Can you work these out from the model? Positions are in its coordinate system, mm. Face numbers are marked on the shaded views. A direction names the side the tool comes from. Coordinates: 2 decimals unless noted, no trailing zeros. Loops run counter-clockwise (first coordinate to the right, second up) from the corner with the lowest first, then second, coordinate; pieces in that order, holes last. Notation, with made-up numbers: M 46.25,87 L 89.25,87 A21 ccw 89.25,121 Z; hole C 30,0.5 d7. An arc over 180 degrees is marked long. Return JSON: item names as keys, results as strings. Group by question number.
```python
from build123d import *

# Parameters (mm, degrees)
SKETCH1_W            = 93
SKETCH1_H            = 100
BOSS_EXTRUDE2_DEPTH  = 10
SKETCH4_W            = 10.01
SKETCH4_H            = 15
BOSS_EXTRUDE4_DEPTH  = 24
SKETCH5_R            = 2
CUT_EXTRUDE1_DEPTH   = 50
SKETCH7_R            = 11
CUT_EXTRUDE3_DEPTH   = 50
SKETCH14_W           = 61.5
SKETCH14_H           = 42
CUT_EXTRUDE8_DEPTH   = 4
SKETCH19_R           = 11
CUT_EXTRUDE11_DEPTH  = 15
SKETCH20_R           = 2
CUT_EXTRUDE12_DEPTH  = 10
SKETCH21_W           = 40
SKETCH21_H           = 6
BOSS_EXTRUDE5_DEPTH  = 27
SKETCH22_W           = 40
SKETCH22_H           = 6.3
BOSS_EXTRUDE7_DEPTH  = 40
SKETCH23_R           = 8
CUT_EXTRUDE13_DEPTH  = 40
SKETCH24_W           = 118.277817783
SKETCH24_H           = 41.8
CUT_EXTRUDE14_DEPTH  = 40
SKETCH25_W           = 31.5
SKETCH25_H           = 23.2
CUT_EXTRUDE15_DEPTH  = 20
CUT_EXTRUDE18_DEPTH  = 3
SKETCH27_R           = 4.1
SKETCH27_R_2         = 4
CUT_EXTRUDE29_DEPTH  = 3
SKETCH28_W           = 29.5
SKETCH28_H           = 58.2
CUT_EXTRUDE30_DEPTH  = 23
SKETCH29_W           = 32
SKETCH29_H           = 4
CUT_EXTRUDE31_DEPTH  = 23
SKETCH31_W           = 32
SKETCH31_H           = 6
BOSS_EXTRUDE9_DEPTH  = 6.6
SKETCH32_W           = 32
SKETCH32_H           = 6
BOSS_EXTRUDE10_DEPTH = 10
SKETCH33_R           = 2
CUT_EXTRUDE32_DEPTH  = 10
BOSS_EXTRUDE11_START = -32
BOSS_EXTRUDE11_DEPTH = 32
SKETCH35_R           = 3.5
CUT_EXTRUDE33_DEPTH  = 10
SKETCH36_W           = 27
SKETCH36_H           = 46
CUT_EXTRUDE34_DEPTH  = 50
SKETCH38_W           = 31.75
SKETCH38_H           = 35
CUT_EXTRUDE35_DEPTH  = 50
SKETCH40_W           = 4
SKETCH40_H           = 77.818306413
CUT_EXTRUDE37_DEPTH  = 110
SKETCH41_W           = 28
SKETCH41_H           = 1.72
CUT_EXTRUDE38_DEPTH  = 50


with BuildPart() as part:
    # Sketch1 → Boss-Extrude2 (new body)
    with BuildSketch(Plane.XY):
        with Locations((-29.68705036, 14.928057554)):
            Rectangle(SKETCH1_W, SKETCH1_H)
    extrude(amount=BOSS_EXTRUDE2_DEPTH)

    # Sketch4 → Boss-Extrude4 (add)
    with BuildSketch(Plane(origin=(16.81294964, 0, 0), x_dir=(0, 0, -1), z_dir=(1, 0, 0))):
        with Locations((-4.995, -12.571942446)):
            Rectangle(SKETCH4_W, SKETCH4_H)
    extrude(amount=BOSS_EXTRUDE4_DEPTH)

    # Sketch5 → Cut-Extrude1 (cut)
    with BuildSketch(Plane(origin=(0, -5.071942446, 0), x_dir=(1, 0, 0), z_dir=(0, 1, 0))):
        with Locations(Location((26.81294964, -5, 0), (0, 0, 180))):
            Circle(SKETCH5_R)
    extrude(amount=-CUT_EXTRUDE1_DEPTH, mode=Mode.SUBTRACT)

    # Sketch7 → Cut-Extrude3 (cut)
    with BuildSketch(Plane(origin=(0, 0, 0), x_dir=(-1, 0, 0), z_dir=(0, 0, -1))):
        with Locations((24.18705036, 36.928057554)):
            Circle(SKETCH7_R)
    extrude(amount=-CUT_EXTRUDE3_DEPTH, mode=Mode.SUBTRACT)

    # Sketch14 → Cut-Extrude8 (cut)
    with BuildSketch(Plane.XY.offset(10)):
        with Locations((-13.93705036, 36.789132279)):
            Rectangle(SKETCH14_W, SKETCH14_H)
    extrude(amount=-CUT_EXTRUDE8_DEPTH, mode=Mode.SUBTRACT)

    # Sketch19 → Cut-Extrude11 (cut)
    with BuildSketch(Plane(origin=(0, 0, 0), x_dir=(-1, 0, 0), z_dir=(0, 0, -1))):
        with Locations((53.18705036, 36.928057554)):
            Circle(SKETCH19_R)
    extrude(amount=-CUT_EXTRUDE11_DEPTH, mode=Mode.SUBTRACT)

    # Sketch20 → Cut-Extrude12 (cut)
    with BuildSketch(Plane.XY.offset(6)):
        with Locations((-34.68705036, 50.928057554)):
            Circle(SKETCH20_R)
        with Locations((5.31294964, 50.928057554)):
            Circle(SKETCH20_R)
        with Locations((-34.68705036, 22.928057554)):
            Circle(SKETCH20_R)
        with Locations((5.31294964, 22.928057554)):
            Circle(SKETCH20_R)
    extrude(amount=-CUT_EXTRUDE12_DEPTH, mode=Mode.SUBTRACT)

    # Sketch21 → Boss-Extrude5 (add)
    with BuildSketch(Plane(origin=(0, 0, 0), x_dir=(-1, 0, 0), z_dir=(0, 0, -1))):
        with Locations((56.18705036, 61.928057554)):
            Rectangle(SKETCH21_W, SKETCH21_H)
    extrude(amount=BOSS_EXTRUDE5_DEPTH)

    # Sketch22 → Boss-Extrude7 (add)
    with BuildSketch(Plane.XZ.offset(-58.928057554)):
        with Locations((-56.18705036, -23.85)):
            Rectangle(SKETCH22_W, SKETCH22_H)
    extrude(amount=BOSS_EXTRUDE7_DEPTH)

    # Sketch23 → Cut-Extrude13 (cut)
    with BuildSketch(Plane.XY.offset(10)):
        with Locations((-53.18705036, 36.928057554)):
            Circle(SKETCH23_R)
    extrude(amount=-CUT_EXTRUDE13_DEPTH, mode=Mode.SUBTRACT)

    # Sketch24 → Cut-Extrude14 (cut)
    with BuildSketch(Plane.XY.offset(10)):
        with Locations((-17.048141468, -14.171942446)):
            Rectangle(SKETCH24_W, SKETCH24_H)
    extrude(amount=-CUT_EXTRUDE14_DEPTH, mode=Mode.SUBTRACT)

    # Sketch25 → Cut-Extrude15 (cut)
    with BuildSketch(Plane.XY.offset(10)):
        with Locations((-60.43705036, 18.328057554)):
            Rectangle(SKETCH25_W, SKETCH25_H)
    extrude(amount=-CUT_EXTRUDE15_DEPTH, mode=Mode.SUBTRACT)

    # Sketch26 → Cut-Extrude18 (cut)
    with BuildSketch(Plane.XY.offset(6)):
        with BuildLine():
            Line((14.30212304, 57.789132279), (6.863398886, 57.789132279))
            Line((6.863398886, 57.789132279), (6.863398886, 54.615347499))
            ThreePointArc((6.863398886, 54.615347499), (8.24773413, 53.645968516), (9.108195728, 52.191428892))
            Line((9.108195728, 52.191428892), (14.30212304, 52.191428892))
            Line((14.30212304, 52.191428892), (14.30212304, 57.789132279))
        make_face()
        with BuildLine():
            Line((6.863398886, 19.240767609), (6.863398886, 15.789132279))
            Line((6.863398886, 15.789132279), (14.30212304, 15.789132279))
            Line((14.30212304, 15.789132279), (14.30212304, 20.928057554))
            Line((14.30212304, 20.928057554), (8.777051255, 20.928057554))
            ThreePointArc((8.777051255, 20.928057554), (7.95835451, 19.927752057), (6.863398886, 19.240767609))
        make_face()
        with BuildLine():
            Line((-36.237499605, 57.789132279), (-44.68705036, 57.789132279))
            Line((-44.68705036, 57.789132279), (-44.68705036, 52.191428892))
            Line((-44.68705036, 52.191428892), (-38.482296447, 52.191428892))
            ThreePointArc((-38.482296447, 52.191428892), (-37.621834849, 53.645968516), (-36.237499605, 54.615347499))
            Line((-36.237499605, 54.615347499), (-36.237499605, 57.789132279))
        make_face()
        with BuildLine():
            Line((-44.68705036, 21.664686216), (-44.68705036, 15.789132279))
            Line((-44.68705036, 15.789132279), (-36.237499605, 15.789132279))
            Line((-36.237499605, 15.789132279), (-36.237499605, 19.240767609))
            ThreePointArc((-36.237499605, 19.240767609), (-37.621834849, 20.210146592), (-38.482296447, 21.664686216))
            Line((-38.482296447, 21.664686216), (-44.68705036, 21.664686216))
        make_face()
    extrude(amount=-CUT_EXTRUDE18_DEPTH, mode=Mode.SUBTRACT)

    # Sketch27 → Cut-Extrude29 (cut)
    with BuildSketch(Plane.XY.offset(6)):
        with Locations((5.31294964, 50.928057554)):
            Circle(SKETCH27_R)
        with Locations((5.31294964, 22.928057554)):
            Circle(SKETCH27_R_2)
        with Locations((-34.68705036, 50.928057554)):
            Circle(SKETCH27_R)
        with Locations((-34.68705036, 22.928057554)):
            Circle(SKETCH27_R)
    extrude(amount=-CUT_EXTRUDE29_DEPTH, mode=Mode.SUBTRACT)

    # Sketch28 → Cut-Extrude30 (cut)
    with BuildSketch(Plane(origin=(0, 0, 0), x_dir=(-1, 0, 0), z_dir=(0, 0, -1))):
        with Locations((-2.06294964, 35.828057554)):
            Rectangle(SKETCH28_W, SKETCH28_H)
    extrude(amount=-CUT_EXTRUDE30_DEPTH, mode=Mode.SUBTRACT)

    # Sketch29 → Cut-Extrude31 (cut)
    with BuildSketch(Plane(origin=(0, 15.789132279, 0), x_dir=(1, 0, 0), z_dir=(0, 1, 0))):
        with Locations((-28.68705036, -8)):
            Rectangle(SKETCH29_W, SKETCH29_H)
    extrude(amount=-CUT_EXTRUDE31_DEPTH, mode=Mode.SUBTRACT)

    # Sketch31 → Boss-Extrude9 (add)
    with BuildSketch(Plane.XZ.offset(-6.728057554)):
        with Locations((-28.68705036, 3)):
            Rectangle(SKETCH31_W, SKETCH31_H)
    extrude(amount=BOSS_EXTRUDE9_DEPTH)

    # Sketch32 → Boss-Extrude10 (add)
    with BuildSketch(Plane.XY.offset(6)):
        with Locations((-28.68705036, 3.128057554)):
            Rectangle(SKETCH32_W, SKETCH32_H)
    extrude(amount=BOSS_EXTRUDE10_DEPTH)

    # Sketch33 → Cut-Extrude32 (cut)
    with BuildSketch(Plane(origin=(0, 6.128057554, 0), x_dir=(1, 0, 0), z_dir=(0, 1, 0))):
        with Locations(Location((-33.68705036, -11, 0), (0, 0, 270))):
            Circle(SKETCH33_R)
        with Locations(Location((-19.68705036, -11, 0), (0, 0, 270))):
            Circle(SKETCH33_R)
    extrude(amount=-CUT_EXTRUDE32_DEPTH, mode=Mode.SUBTRACT)

    # Sketch34 → Boss-Extrude11 (add)
    with BuildSketch(Plane(origin=(-12.68705036, 0, 0), x_dir=(0, 0, -1), z_dir=(1, 0, 0)).offset(BOSS_EXTRUDE11_START)):
        Polygon((-16, 6.128057554), (-6, 6.128057554), (-6, 14.058360342), align=None)
    extrude(amount=BOSS_EXTRUDE11_DEPTH)

    # Sketch35 → Cut-Extrude33 (cut)
    with BuildSketch(Plane.XZ.offset(-6.128057554)):
        with Locations((-19.68705036, 11)):
            Circle(SKETCH35_R)
        with Locations((-33.68705036, 11)):
            Circle(SKETCH35_R)
    extrude(amount=-CUT_EXTRUDE33_DEPTH, mode=Mode.SUBTRACT)

    # Sketch36 → Cut-Extrude34 (cut)
    with BuildSketch(Plane(origin=(-36.18705036, 0, 0), x_dir=(0, 0, -1), z_dir=(1, 0, 0))):
        with Locations((13.5, 41.928057554)):
            Rectangle(SKETCH36_W, SKETCH36_H)
    extrude(amount=-CUT_EXTRUDE34_DEPTH, mode=Mode.SUBTRACT)

    # Sketch38 → Cut-Extrude35 (cut)
    with BuildSketch(Plane.XY.offset(10)):
        with Locations((-60.31205036, 47.428057554)):
            Rectangle(SKETCH38_W, SKETCH38_H)
    extrude(amount=-CUT_EXTRUDE35_DEPTH, mode=Mode.SUBTRACT)

    # Sketch40 → Cut-Extrude37 (cut)
    with BuildSketch(Plane.XY.offset(16)):
        with Locations((-42.68705036, 39.037210761)):
            Rectangle(SKETCH40_W, SKETCH40_H)
    extrude(amount=-CUT_EXTRUDE37_DEPTH, mode=Mode.SUBTRACT)

    # Sketch41 → Cut-Extrude38 (cut)
    with BuildSketch(Plane.XY.offset(16)):
        with Locations((-26.68705036, 0.988057554)):
            Rectangle(SKETCH41_W, SKETCH41_H)
    extrude(amount=-CUT_EXTRUDE38_DEPTH, mode=Mode.SUBTRACT)


solid = part.part
```
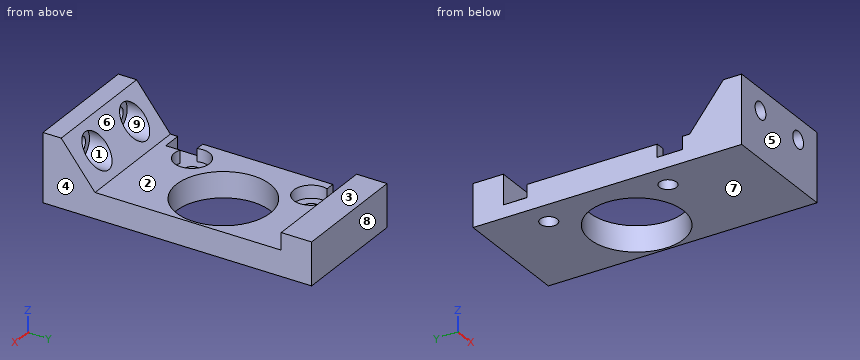
1) For the marked faces 1, 2, 3, 4 and 5, which set-ups out of +Z, -Z, +X, -X, +Y, -Y let a thin tool reach every point of the face, with its end or its side?
2) Suppose I cut it at C-C, the plane z = 8.25. List the corners of the cut face in (x, y) for me.
3) For pin 1 (8 mm diameter, centred on x = -37.5, y = 22.5, fed in from +Z); pin 2 (2.5 mm diameter, centred on x = -34.69, y = 50.93, fed in from +Z); pin 3 (0.9 mm diameter, centred on y = 17.5, z = 4.5, fed in from -X); pin 4 (5.5 mm diameter, centred on x = -30, y = 62, fed in from +Z), each with a flat end and sliding along its axis, tell me the tip position at first contact or that it passes through.
4) Suppose I cut it at A-A, the plane y = 41. List the corners of the cut face in (x, z) for me, then the cut area to 3 significant figures.
5) If I drill on line 1 (X direction, y = 3.3, z = 11); line 2 (Y direction, x = -36.5, z = 1.75); line 3 (Z direction, x = -36.75, y = 33), over which ranges is the centre line in solid material (lowest first)? Write a range as from..to.
6) If we mould it in two halves opening along Z, with no side actions, what happens to the marked faces 6, 7, 8 and 9? For each: +Z half, -Z half, draft (parallel to the pull), parting line (faces both ways), or undercut.
7) Suppose I cut it at D-D, the plane z = 11. List the corners of the cut face in (x, y) for me, then the cut area to 3 significant figures.
8) Suppose I cut it at B-B, the plane x = -27.75. List the corners of the cut face in (y, z) for me.
Returned:
{
 "1": {"face 1": "none", "face 2": "+Z, +X, -X", "face 3": "+Z, +X, -X, +Y", "face 4": "+Z, -Z, +X, +Y, -Y", "face 5": "+Z, -Z, +X, -X, -Y"},
 "2": {"outline": "M -40.69,1.85 L -12.69,1.85 L -12.69,12.27 L -17.52,12.27 L -17.52,6.13 L -21.85,6.13 L -21.85,12.27 L -31.52,12.27 L -31.52,6.13 L -35.85,6.13 L -35.85,12.27 L -40.69,12.27 Z; M -40.69,57.79 L -12.69,57.79 L -12.69,64.93 L -40.69,64.93 Z"},
 "3": {"pin 1": "stops at z = 6", "pin 2": "passes through", "pin 3": "stops at x = -36.24", "pin 4": "stops at z = 10"},
 "4": {"outline": "M -40.69,0 L -34.41,0 L -34.41,6 L -40.69,6 Z; M -13.97,0 L -12.69,0 L -12.69,6 L -13.97,6 Z", "area": "45.4 mm²"},
 "5": {"line 1": "x = -40.69..-35.69, -31.69..-21.69, -17.69..-12.69", "line 2": "y = 1.85..22.08, 23.77..50.08, 51.77..64.93", "line 3": "z = 0..6"},
 "6": {"face 6": "+Z half", "face 7": "-Z half", "face 8": "draft", "face 9": "undercut"},
 "7": {"outline": "M -40.69,1.85 L -35.69,1.85 L -35.69,6.13 L -37.19,6.13 L -37.19,10.09 L -40.69,10.09 Z; M -31.69,1.85 L -21.69,1.85 L -21.69,6.13 L -23.19,6.13 L -23.19,10.09 L -30.19,10.09 L -30.19,6.13 L -31.69,6.13 Z; M -17.69,1.85 L -12.69,1.85 L -12.69,10.09 L -16.19,10.09 L -16.19,6.13 L -17.69,6.13 Z", "area": "141 mm²"},
 "8": {"outline": "M 1.85,0 L 26.52,0 L 26.52,6 L 14.06,6 L 6.13,16 L 1.85,16 Z; M 47.34,0 L 64.93,0 L 64.93,10 L 57.79,10 L 57.79,6 L 47.34,6 Z"}
}
